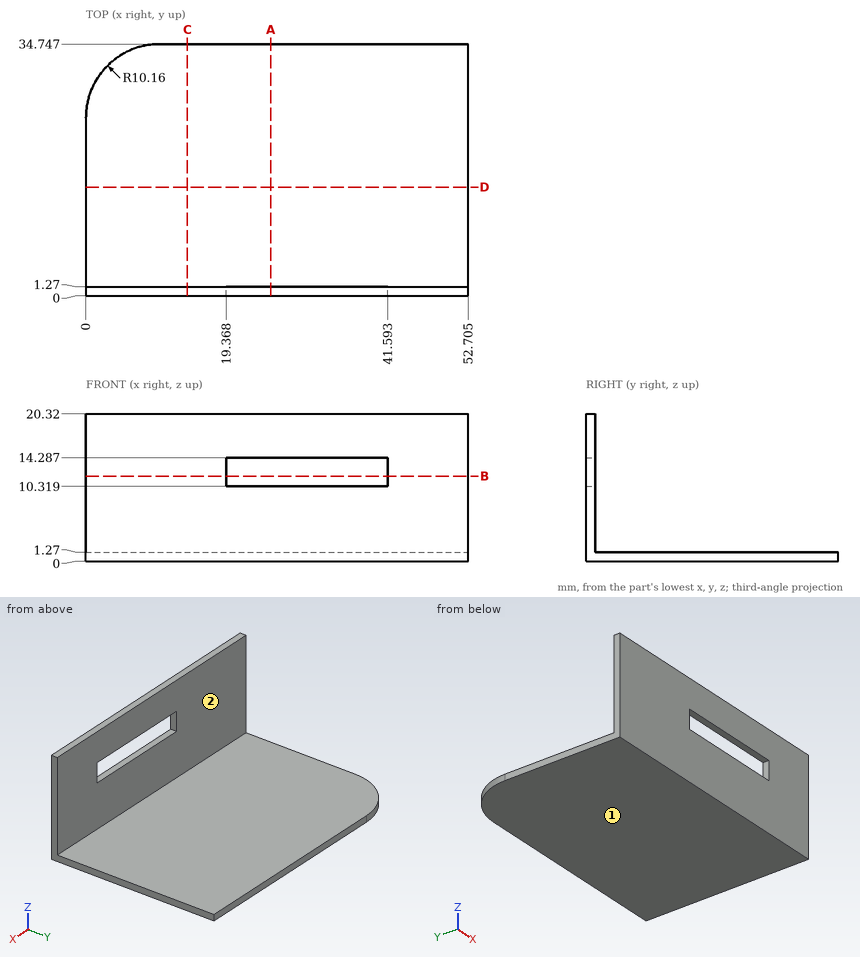
Could you check a few things on this drawing? It's one solid part, dimensions in mm from its lowest x, y, z. A direction names the side the tool comes from. Give positions to 0.01 mm unless a question says otherwise; leave off trailing zeros. Order: outer loops, then holes, each group sorted by start corner. A loop starts at its lowest first (then second) coordinate and runs counter-clockwise, first axis right, second up. Notation, with made-up numbers: (-23, 82.5) - (5, 82.5) arc R25 ccw to (5, 103.5) - close; hole circle Ø7 at (56, 83.25). An arc over 180 degrees is marked (long way). Answer as a JSON object with one key per item and string values. Group by question number.
Item 1: If we section it at A-A on x = 25.5: Please give me the cut outline in (y, z).
Item 2: If we section it at D-D on y = 15: Please give me the cut outline in (x, z) (1 decimal).
Item 3: Which directions (+Z, -Z, +X, -X, +Y, -Y) give clear straight access to the entire face, cutting with the end or side of a thin tool? Please do the marked faces 1 and 2.
Item 4: If we section it at B-B on z = 11.75: Please give me the cut outline in (x, y) (1 decimal).
Item 5: Please list where this line runs through material, in increasing order: probe 1 along Y at (x, z) = (34, 9).
Item 6: For P1, Ø4, axis at x = 8, y = 21.5, coming from the +Z side; P2, Ø12, axis at y = 10, z = 14.5, coming from the +X side; P3, Ø9.5, axis at x = 15, z = 14.5, coming from the +Y side, each with a flat end and sliding along its axis, tell me the tip position at first contact or that it passes through.
Item 7: If we section it at C-C on x = 14: Please give me the cut outline in (y, z).
Result set:
{
 "1": {"outline": "(0, 0) - (34.75, 0) - (34.75, 1.27) - (1.27, 1.27) - (1.27, 10.32) - (0, 10.32) - close; (0, 14.29) - (1.27, 14.29) - (1.27, 20.32) - (0, 20.32) - close"},
 "2": {"outline": "(0, 0) - (52.7, 0) - (52.7, 1.3) - (0, 1.3) - close"},
 "3": {"face 1": "-Z, +X, -X, +Y, -Y", "face 2": "+Z, +X, -X, +Y"},
 "4": {"outline": "(0, 0) - (19.4, 0) - (19.4, 1.3) - (0, 1.3) - close; (41.6, 0) - (52.7, 0) - (52.7, 1.3) - (41.6, 1.3) - close"},
 "5": {"probe 1": "0 to 1.27"},
 "6": {"P1": "z = 1.27", "P2": "through", "P3": "y = 1.27"},
 "7": {"outline": "(0, 0) - (34.75, 0) - (34.75, 1.27) - (1.27, 1.27) - (1.27, 20.32) - (0, 20.32) - close"}
}
